Work out the finished part from the listing and answer in its coordinate system (mm). Face numbers are marked on the shaded views. A direction names the side the tool comes from. Give positions to 0.01 mm unless a question says otherwise; leave off trailing zeros. Write each loop counter-clockwise with the first axis right and the second up, starting at its lowest first coordinate (ties: lowest second). Pieces come first, ordered by that corner, then holes. Notation, with made-up numbers: (84.25, -8.5) - (91.25, -8.5) arc R30 ccw to (91.25, 26.5) - close; hole circle Ø4 at (-20, -3). An arc over 180 degrees is marked (long way). Write item = value, one per line.
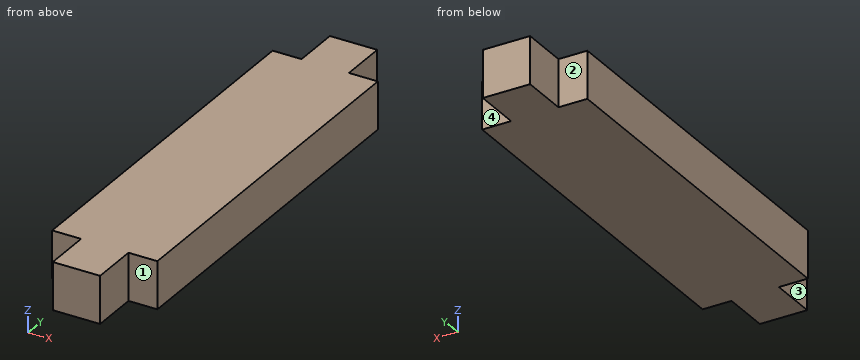
from build123d import *

# Parameters (mm, degrees)
SKETCH2_W           = 4.5
SKETCH2_H           = 4.5
SKETCH2_W_2         = 10
SKETCH2_H_2         = 17.5
BOSS_EXTRUDE1_DEPTH = 2.25


with BuildPart() as part:
    # Sketch2 → Boss-Extrude1 (new body, symmetric)
    with BuildSketch(Plane.XY):
        with Locations((0, 19.75)):
            Rectangle(SKETCH2_W, SKETCH2_H)
        with Locations((0, 8.75)):
            Rectangle(SKETCH2_W_2, SKETCH2_H_2)
    extrude(amount=BOSS_EXTRUDE1_DEPTH, both=True)

    # Mirror1: part across plane


with BuildPart() as part_1:
    add(part.part)
    add(part.part.mirror(Plane.ZX))


solid = part_1.part
1. Find section B-B, the plane x = -4.5. Give the vertices of the cut face in (y, z).
Solution:
outline = (-17.5, -2.25) - (17.5, -2.25) - (17.5, 2.25) - (-17.5, 2.25) - close
2. Find section A-A, the plane z = 1.15. Give the vertices of the cut face in (x, y), then the cut area to 4 significant figures.
Solution:
outline = (-5, -17.5) - (-2.25, -17.5) - (-2.25, -22) - (2.25, -22) - (2.25, -17.5) - (5, -17.5) - (5, 17.5) - (2.25, 17.5) - (2.25, 22) - (-2.25, 22) - (-2.25, 17.5) - (-5, 17.5) - close
area = 390.5 mm^2
3. Given pin 1 (0.8 mm diameter, centred on x = -3, z = 0.5, fed in from -Y); pin 2 (1.3 mm diameter, centred on y = 18.5, z = 1, fed in from +X); pin 3 (1.3 mm diameter, centred on y = -20, z = 0.5, fed in from -X), each flat-ended and moving along its own axis, determine where each tip first touches the part or whether it passes through.
Solution:
pin_1 = -17.5
pin_2 = 2.25
pin_3 = -2.25
4. Straight lines are drawn through the part: line 1 (Y direction, x = 3.5, z = 0.1); line 2 (X direction, y = 20, z = 0.65). For each, find the intervals that lie inside material, in ascending order.
Solution:
line_1 = -17.5 to 17.5
line_2 = -2.25 to 2.25
5. A tool of negligible diameter and unlimited length cuts with its end or side. For the marked faces 1, 2, 3 and 4, from which of +Z, -Z, +X, -X, +Y, -Y can it reach the whole face along a straight path? Write none if from no direction.
Solution:
face_1 = +Z, -Z, +X, -Y
face_2 = +Z, -Z, -X, +Y
face_3 = +Z, -Z, -X, -Y
face_4 = +Z, -Z, +X, +Y
